```python
from build123d import *

# Parameters (mm, degrees)
BOSS_EXTRUDE4_DEPTH = 80
BOSS_EXTRUDE5_DEPTH = 57
CUT_EXTRUDE1_DEPTH  = 3
SKETCH13_W          = 46.599854234
SKETCH13_H          = 36.724502986
CUT_EXTRUDE2_DEPTH  = 45


with BuildPart() as part:
    # Sketch8 → Boss-Extrude4 (new body)
    with BuildSketch(Plane(origin=(0, 58, 0), x_dir=(1, 0, 0), z_dir=(0, 1, 0))):
        with BuildLine():
            Line((-11.242998334, -12), (11.242998334, -12))
            ThreePointArc((11.242998334, -12), (14.65898123, -10.932652517), (16.859617211, -8.110353618))
            add(Edge.make_bspline(
                [(16.859617211, -8.110353618), (17.850691543, -5.472650271), (18.834301198, 0.028433299), (17.819526576, 5.426475932), (16.811684839, 8.109721769)],
                knots=[0.167422492, 0.167422492, 0.167422492, 0.167422492, 0.502499344, 0.837905074, 0.837905074, 0.837905074, 0.837905074], degree=3))
            ThreePointArc((16.811684839, 8.109721769), (14.611088933, 10.932460371), (11.194828596, 12))
            Line((11.194828596, 12), (-11.194828596, 12))
            ThreePointArc((-11.194828596, 12), (-14.611088933, 10.932460371), (-16.811684839, 8.109721769))
            add(Edge.make_bspline(
                [(-16.859617211, -8.110353618), (-17.850691543, -5.472650271), (-18.834301198, 0.028433299), (-17.819526576, 5.426475932), (-16.811684839, 8.109721769)],
                knots=[0.167422492, 0.167422492, 0.167422492, 0.167422492, 0.502499344, 0.837905074, 0.837905074, 0.837905074, 0.837905074], degree=3))
            ThreePointArc((-16.859617211, -8.110353618), (-14.65898123, -10.932652517), (-11.242998334, -12))
        make_face()
        with BuildLine():
            Line((-13, -10), (13, -10))
            ThreePointArc((13, -10), (14.414213562, -9.414213562), (15, -8))
            Line((15, -8), (15, 8))
            ThreePointArc((15, 8), (14.414213562, 9.414213562), (13, 10))
            Line((13, 10), (-13, 10))
            ThreePointArc((-13, 10), (-14.414213562, 9.414213562), (-15, 8))
            Line((-15, 8), (-15, -8))
            ThreePointArc((-15, -8), (-14.414213562, -9.414213562), (-13, -10))
        make_face(mode=Mode.SUBTRACT)
    extrude(amount=BOSS_EXTRUDE4_DEPTH)

    # Sketch11 → Boss-Extrude5 (add)
    with BuildSketch(Plane(origin=(0, 58, 0), x_dir=(1, 0, 0), z_dir=(0, 1, 0))):
        with BuildLine():
            Line((13, 10), (15, 10))
            Line((15, 10), (15, 6.937911183))
            Line((15, 6.937911183), (13.5, 6.937911183))
            ThreePointArc((13.5, 6.937911183), (13.146446609, 7.084357793), (13, 7.437911183))
            Line((13, 7.437911183), (13, 10))
        make_face()
        with BuildLine():
            Line((-13, 7.437911183), (-13, 10))
            Line((-13, 10), (-15, 10))
            Line((-15, 10), (-15, 6.937911183))
            Line((-15, 6.937911183), (-13.5, 6.937911183))
            ThreePointArc((-13.5, 6.937911183), (-13.146446609, 7.084357793), (-13, 7.437911183))
        make_face()
    extrude(amount=BOSS_EXTRUDE5_DEPTH)

    # Sketch12 → Cut-Extrude1 (cut)
    with BuildSketch(Plane.XY.offset(12)):
        with BuildLine():
            Line((7.476357736, 134.986611492), (7.476357736, 114.986611492))
            ThreePointArc((7.476357736, 114.986611492), (-0.023642264, 107.486611492), (-7.523642264, 114.986611492))
            Line((-7.523642264, 114.986611492), (-7.523642264, 134.986611492))
            Line((-7.523642264, 134.986611492), (-8.023642264, 134.986611492))
            Line((-8.023642264, 134.986611492), (-8.023642264, 114.986611492))
            ThreePointArc((-8.023642264, 114.986611492), (-0.023642264, 106.986611492), (7.976357736, 114.986611492))
            Line((7.976357736, 114.986611492), (7.976357736, 134.986611492))
            Line((7.976357736, 134.986611492), (7.476357736, 134.986611492))
        make_face()
    extrude(amount=-CUT_EXTRUDE1_DEPTH, mode=Mode.SUBTRACT)

    # Sketch13 → Cut-Extrude2 (cut)
    with BuildSketch(Plane(origin=(0, 58, 0), x_dir=(1, 0, 0), z_dir=(0, 1, 0))):
        with Locations((3.699497448, 5.974004227)):
            Rectangle(SKETCH13_W, SKETCH13_H)
    extrude(amount=CUT_EXTRUDE2_DEPTH, mode=Mode.SUBTRACT)


solid = part.part
```
Work out the finished part from the listing and answer in its coordinate system (mm). A direction names the side the tool comes from. Give positions to 0.01 mm unless a question says otherwise; leave off trailing zeros. Order: outer loops, then holes, each group sorted by start corner. A loop starts at its lowest first (then second) coordinate and runs counter-clockwise, first axis right, second up.
1. Section A-A, the plane x = -6.5 is taken. Determine the outline of the cut face in (y, z).
Result sheet:
outline: (103, -12) - (138, -12) - (138, -10) - (103, -10) - close; (103, 10) - (110.29, 10) - (110.29, 12) - (103, 12) - close; (111.2, 10) - (138, 10) - (138, 12) - (111.2, 12) - close
2. Section B-B, the plane z = 10.75 is taken. Determine the outline of the cut face in (x, y), and give its area (3 significant figures).
Result sheet:
outline: (-14.91, 103) - (14.91, 103) - (14.91, 138) - (-14.91, 138) - close; hole (-8.02, 114.99) arc R8 ccw to (7.98, 114.99) - (7.98, 134.99) - (7.48, 134.99) - (7.48, 114.99) arc R7.5 cw to (-7.52, 114.99) - (-7.52, 134.99) - (-8.02, 134.99) - close
area: 1,010 mm2
3. Section C-C, the plane x = 12 is taken. Determine the outline of the cut face in (y, z).
Result sheet:
outline: (103, -11.95) - (138, -11.95) - (138, -10) - (103, -10) - close; (103, 10) - (138, 10) - (138, 11.95) - (103, 11.95) - close
4. The mould has two halves that part along Y. Classify faces 1 (the flat face through (14, 115, -8)), 2 (the flat face through (7.976, 125, 11)), 3 (the flat face through (13, 109, -9)), 4 (the flat face through (-7.524, 125, 11)): released by +Y, released by -Y, zero draft, split by the parting line, or undercut.
Result sheet:
face 1: released by +Y
face 2: undercut
face 3: zero draft
face 4: undercut
5. Each of these flat-tipped pins is pushed along its axis until it touches: P1, Ø6, axis at y = 116.5, z = -8, coming from the +X side; P2, Ø4, axis at y = 127.5, z = -9, coming from the +X side; P3, Ø12, axis at y = 130, z = 6.5, coming from the +X side. Where does it stop, or does it pass through?
Result sheet:
P1: stops at x = 17.75
P2: stops at x = 17.2
P3: stops at x = 18.33
6. For faces 5 (the cylindrical face through (0.14, 107.49, 11.01)), 6 (the cylindrical face through (-14.43, 120.26, 9.4)), 7 (the flat face through (-14, 115, -8)), 8 (the cylindrical face through (14.62, 120.26, 10.96)), determine the directions among +Z, -Z, +X, -X, +Y, -Y from which every point of the face is accessible in a straight line to the end or side of a thin tool.
Result sheet:
face 5: +Z
face 6: +Y, -Y
face 7: +Y
face 8: +Z, +X, +Y, -Y
7. Straight lines are drawn through the part: L1, parallel to Z at x = 11.5, y = 133.5; L2, parallel to X at y = 125, z = -0.25; L3, parallel to X at y = 111, z = -3.25. For each, find the intervals that lie inside material, in ascending order.
Result sheet:
L1: z = -11.99 to -10, 10 to 11.99
L2: x = -18.33 to -15, 15 to 18.33
L3: x = -18.09 to -15, 15 to 18.09
